```python
from build123d import *

# Parameters (mm, degrees)
F0_W        = 5
F0_H        = 10
F1_DEPTH    = 20
F2_T1_DEPTH = 45
F3_R        = 2.5
F4_DEPTH    = 25


# Not quite as in the source:
# - a fillet or chamfer that OpenCascade refuses, or shapes differently, is made with other operations: its cross-section is extruded or revolved along the edge and cut away or added


with BuildPart() as f1:
    # F0 (on Front) → F1 (new body)
    with BuildSketch(Plane.XZ):
        Rectangle(F0_W, F0_H)
    extrude(amount=F1_DEPTH)

    # F2: fillet of radius 5 on 2 edges, made by hand

    # F2_s2 → F2_t1 (cut)
    with BuildSketch(Plane.XZ.offset(-12.5)):
        with BuildLine():
            ThreePointArc((-2.5, 0), (-1.0355339059, -3.5355339059), (2.5, -5))
            Line((2.5, -5), (-2.5, -5))
            Line((-2.5, -5), (-2.5, 0))
        make_face()
        with BuildLine():
            ThreePointArc((-2.5, -5), (1.0355339059, -3.5355339059), (2.5, 0))
            Line((2.5, 0), (2.5, -5))
            Line((2.5, -5), (-2.5, -5))
        make_face()
    extrude(amount=F2_T1_DEPTH, mode=Mode.SUBTRACT)

    # F3 (on face) → F4 (join)
    with BuildSketch(Plane.XY.offset(5)):
        with Locations((0, -10)):
            Circle(F3_R)
    extrude(amount=F4_DEPTH)


solid = f1.part
```
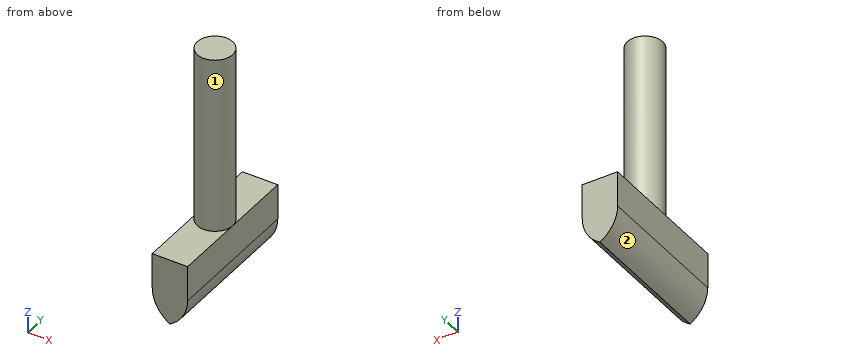
Design review of the part built by this model. Coordinates are the model's own, in mm. Face numbers are marked on the shaded views. A direction names the side the tool comes from. Coordinates: 2 decimals unless noted, no trailing zeros. Order: outer loops, then holes, each group sorted by start corner. A loop starts at its lowest first (then second) coordinate and runs counter-clockwise, first axis right, second up.
1) Clearance check with flat-ended pins moving along their axes: pin 1 (2 mm diameter, centred on x = -0.5, z = 18.5, fed in from -Y); pin 2 (1 mm diameter, centred on x = -2, y = -12, fed in from -Z); pin 3 (2.5 mm diameter, centred on x = 1, y = -4, fed in from +Z). State where each tip first meets the part, or that it passes through.
2) Take a section at D-D, the plane x = -0.45. Give the boundary of the cut face in (y, z), and give its area (3 significant figures).
3) Wall thickness on line 1 along Y through (x, z) = (-0.2, 24.5); line 2 along Z through (x, y) = (-1.5, -18.25); line 3 along Y through (x, z) = (-1.8, 18.5): over which ranges is each line inside the solid? List them lowest first.
4) Take a section at A-A, the plane y = -15. Give the boundary of the cut face in (x, z), and give its area (3 significant figures).
5) Take a section at B-B, the plane x = -1.9. Give the boundary of the cut face in (y, z).
6) Take a section at C-C, the plane z = 14.5. Give the boundary of the cut face in (x, y), and give its area (3 significant figures).
7) For the marked faces 1 and 2, list the 3-axis set-ups (+Z, -Z, +X, -X, +Y, -Y) from which the entire face can be reached by the end or side of a thin tool; tool diameter is ignored.
Returned:
1. pin 1: stops at y = -12.5
1. pin 2: stops at z = -3
1. pin 3: stops at z = 5
2. outline: (-20, -4.04) - (0, -4.04) - (0, 5) - (-7.54, 5) - (-7.54, 30) - (-12.46, 30) - (-12.46, 5) - (-20, 5) - close
2. area: 304 mm2
3. line 1: y = -12.49 to -7.51
3. line 2: z = -3 to 5
3. line 3: y = -11.73 to -8.27
4. outline: (-2.5, 0) arc R5 ccw to (0, -4.33) arc R5 ccw to (2.5, 0) - (2.5, 5) - (-2.5, 5) - close
4. area: 40.4 mm2
5. outline: (-20, -2.37) - (0, -2.37) - (0, 5) - (-8.38, 5) - (-8.38, 30) - (-11.62, 30) - (-11.62, 5) - (-20, 5) - close
6. outline: circle Ø5 at (0, -10)
6. area: 19.6 mm2
7. face 1: +Z
7. face 2: -Z, -X, +Y, -Y
